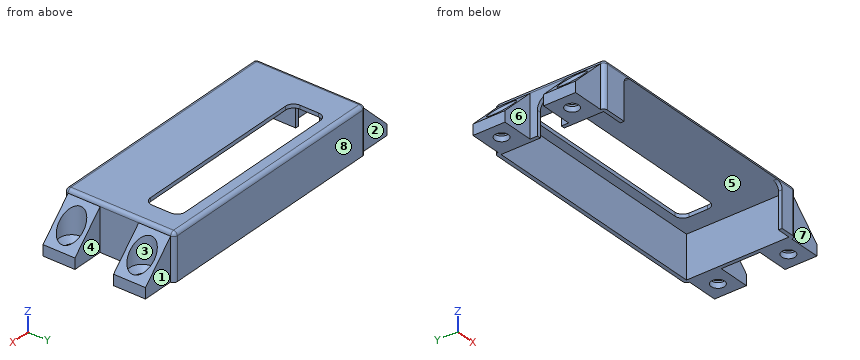
from build123d import *

# Parameters (mm, degrees)
SKETCH_W         = 88.5
SKETCH_H         = 38.5
PAD_DEPTH        = 16
THICKNESS_T      = 1.4
POCKET_DEPTH     = 1.4
POCKET001_DEPTH  = 5
POCKET002_DEPTH  = 5
SKETCH004_W      = 12
SKETCH004_H      = 4
PAD001_DEPTH     = 12
HOLE_D           = 5
HOLE_DEPTH       = 25
HOLE_CSINK_D     = 9
HOLE_CSINK_ANGLE = 90
SKETCH006_W      = 12
SKETCH006_H      = 12
SKETCH006_R      = 4.5
PAD002_DEPTH     = 11.99
POCKET003_DEPTH  = 265.106151


with BuildPart() as part:
    # Sketch → Pad (new body)
    with BuildSketch(Plane.XY):
        with Locations((0, 19.25)):
            Rectangle(SKETCH_W, SKETCH_H)
    extrude(amount=PAD_DEPTH)

    # Thickness
    thickness_openings = [part.faces().sort_by_distance(p)[0] for p in [
        (0, 19.25, 0),
    ]]
    offset(amount=THICKNESS_T, openings=thickness_openings)

    # Sketch001 (on Face14 of Thickness) → Pocket (cut)
    with BuildSketch(Plane(origin=(-45.65, 0, 0), x_dir=(0, -1, 0), z_dir=(-1, 0, 0))):
        with BuildLine():
            Line((-23.75, 0), (-23.75, 9))
            ThreePointArc((-14.75, 9), (-19.25, 13.5), (-23.75, 9))
            Line((-14.75, 0), (-14.75, 9))
            Line((-23.75, 0), (-14.75, 0))
        make_face()
    extrude(amount=-POCKET_DEPTH, mode=Mode.SUBTRACT)

    # Sketch002 (on Face26 of Pocket) → Pocket001 (cut)
    with BuildSketch(Plane.XY.offset(17.4)):
        with BuildLine():
            ThreePointArc((-30.25, 35), (-32.37132, 34.12132), (-33.25, 32))
            Line((-33.25, 25), (-33.25, 32))
            ThreePointArc((-33.25, 25), (-32.37132, 22.87868), (-30.25, 22))
            Line((34.25, 22), (-30.25, 22))
            ThreePointArc((34.25, 22), (36.37132, 22.87868), (37.25, 25))
            Line((37.25, 32), (37.25, 25))
            ThreePointArc((37.25, 32), (36.37132, 34.12132), (34.25, 35))
            Line((-30.25, 35), (34.25, 35))
        make_face()
    extrude(amount=-POCKET001_DEPTH, mode=Mode.SUBTRACT)

    # Sketch003 (on Face16 of Pocket001) → Pocket002 (cut)
    with BuildSketch(Plane.XZ.offset(1.4)):
        with BuildLine():
            Line((39.25, 0), (-36.25, 0))
            Line((-36.25, 0), (-36.25, 13.5))
            ThreePointArc((-33.75, 16), (-35.517767, 15.267767), (-36.25, 13.5))
            Line((-33.75, 16), (36.75, 16))
            ThreePointArc((39.25, 13.5), (38.517767, 15.267767), (36.75, 16))
            Line((39.25, 13.5), (39.25, 0))
        make_face()
    extrude(amount=-POCKET002_DEPTH, mode=Mode.SUBTRACT)

    # Sketch004 (on Face9 of Pocket002) → Pad001 (join)
    with BuildSketch(Plane(origin=(-45.65, 0, 0), x_dir=(0, -1, 0), z_dir=(-1, 0, 0))):
        with Locations((-32.5, 2)):
            Rectangle(SKETCH004_W, SKETCH004_H)
        with Locations((-6, 2)):
            Rectangle(SKETCH004_W, SKETCH004_H)
    pad001 = extrude(amount=PAD001_DEPTH)

    # Hole
    with Locations(Plane.XY.offset(4)):
        with Locations((-51.65, 32.5), (-51.65, 6)):
            hole = CounterSinkHole(HOLE_D / 2, HOLE_CSINK_D / 2, depth=HOLE_DEPTH, counter_sink_angle=HOLE_CSINK_ANGLE)

    # Sketch006 (on Face35 of Hole) → Pad002 (join)
    with BuildSketch(Plane.XY.offset(4)):
        with Locations((-51.65, 6)):
            Rectangle(SKETCH006_W, SKETCH006_H)
        with Locations((-51.65, 6)):
            Circle(SKETCH006_R, mode=Mode.SUBTRACT)
        with Locations((-51.65, 32.5)):
            Rectangle(SKETCH006_W, SKETCH006_H)
        with Locations((-51.65, 32.5)):
            Circle(SKETCH006_R, mode=Mode.SUBTRACT)
    pad002 = extrude(amount=PAD002_DEPTH)

    # Sketch007 (on Face56 of Pad002) → Pocket003 (cut, through all)
    with BuildSketch(Plane(origin=(0, 38.5, 0), x_dir=(-1, 0, 0), z_dir=(0, 1, 0))):
        Polygon((45.65, 15.99), (57.65, 15.99), (57.65, 4), align=None)
    pocket003 = extrude(amount=-POCKET003_DEPTH, mode=Mode.SUBTRACT)

    # Mirrored: Pad001, Hole, Pad002, Pocket003 across YZ
    add(pad001.mirror(Plane.YZ))
    add(hole.mirror(Plane.YZ), mode=Mode.SUBTRACT)
    add(pad002.mirror(Plane.YZ))
    add(pocket003.mirror(Plane.YZ), mode=Mode.SUBTRACT)


solid = part.part
Work out the finished part from the listing and answer in its coordinate system (mm). Face numbers are marked on the shaded views. A direction names the side the tool comes from. Give positions to 0.01 mm unless a question says otherwise; leave off trailing zeros. Order: outer loops, then holes, each group sorted by start corner. A loop starts at its lowest first (then second) coordinate and runs counter-clockwise, first axis right, second up. Notation, with made-up numbers: M -34,83 L -8,83 A23 ccw -8,122 Z; hole C 15.5,-33 d6. An arc over 180 degrees is marked long. Return JSON: item names as keys, results as strings.
Q1. Find section C-C, the plane x = -51.65. Write down the section's boundary in (y, z) (3 decimals).
Answer below:
{"outline": "M 0,0 L 3.5,0 L 3.5,2 L 1.5,4 L 1.5,9.995 L 0,9.995 Z; M 8.5,0 L 12,0 L 12,9.995 L 10.5,9.995 L 10.5,4 L 8.5,2 Z; M 26.5,0 L 30,0 L 30,2 L 28,4 L 28,9.995 L 26.5,9.995 Z; M 35,0 L 38.5,0 L 38.5,9.995 L 37,9.995 L 37,4 L 35,2 Z"}
Q2. Find section A-A, the plane x = 9. Write down the section's boundary in (y, z).
Answer below:
{"outline": "M -1.4,16 L 22,16 L 22,17.4 L 0,17.4 A1.4 ccw Z; M 35,16 L 38.5,16 L 38.5,0 L 39.9,0 L 39.9,16 A1.4 ccw 38.5,17.4 L 35,17.4 Z"}
Q3. Which of the six approach directions +Z, -Z, +X, -X, +Y, -Y give full straight-line access (tool end or side, diameter ignored) to the marked faces 1, 2, 3, 4 and 5?
Answer below:
{"face 1": "+Z, -Z, +X, +Y", "face 2": "+Z, -Z, -X, +Y", "face 3": "+Z", "face 4": "+Z, -Z, +X", "face 5": "-Z"}
Q4. Find the intervals of material crossed by line 1 along Y through (x, z) = (-51.65, 1); line 2 along X through (y, z) = (6, 0.45); line 3 along Y through (x, z) = (51.65, 8), in increasing order. Write a range as [from, to].
Answer below:
{"line 1": "y = [0, 3.5], [8.5, 12], [26.5, 30], [35, 38.5]", "line 2": "x = [-57.65, -54.15], [-49.15, -44.25], [44.25, 49.15], [54.15, 57.65]", "line 3": "y = [0, 1.5], [10.5, 12], [26.5, 28], [37, 38.5]"}
Q5. Each of these flat-tipped pins is pushed along its axis until it touches: pin 1 (4.5 mm diameter, centred on x = -51.65, y = 6, fed in from -Z); pin 2 (1.5 mm diameter, centred on x = 21, y = 10.5, fed in from -Z); pin 3 (9.5 mm diameter, centred on x = -52, z = 10, fed in from +Y); pin 4 (3 mm diameter, centred on y = 26, z = 13, fed in from -X). Where does it stop, or does it pass through?
Answer below:
{"pin 1": "passes through", "pin 2": "stops at z = 16", "pin 3": "stops at y = 38.5", "pin 4": "stops at x = -50.06"}
Q6. Find section B-B, the plane y = 13. Write down the section's boundary in (x, z).
Answer below:
{"outline": "M -45.65,0 L -44.25,0 L -44.25,16 L 44.25,16 L 44.25,0 L 45.65,0 L 45.65,16 A1.4 ccw 44.25,17.4 L -44.25,17.4 A1.4 ccw -45.65,16 Z"}
Q7. Find section D-D, the plane y = 6. State how many separate pieces and enclosed holes the cut face has, and give its area (3 significant figures).
Answer below:
{"separate pieces": "3", "enclosed holes": "0", "area": "256 mm^2"}
Q8. The mould has two halves that part along Y. Classify the marked faces 6, 7 and 8: pulls with the +Y half, pulls with the -Y half, needs draft (parallel to the pull), parting line crosses it, or undercut.
Answer below:
{"face 6": "undercut", "face 7": "pulls with the -Y half", "face 8": "pulls with the +Y half"}
